Read the model definition and answer for the solid it produces. Units are mm, in the model's axes. Face numbers are marked on the shaded views. A direction names the side the tool comes from. Give positions to 0.01 mm unless a question says otherwise; leave off trailing zeros. Write each loop counter-clockwise with the first axis right and the second up, starting at its lowest first coordinate (ties: lowest second). Pieces come first, ordered by that corner, then holes. Notation, with made-up numbers: (3.5, -5) -> (38.5, -5) arc R15 cw to (38.5, 23) -> close; hole circle Ø11 at (-22, -23.5). An arc over 180 degrees is marked (long way). Write item = value, one per line.
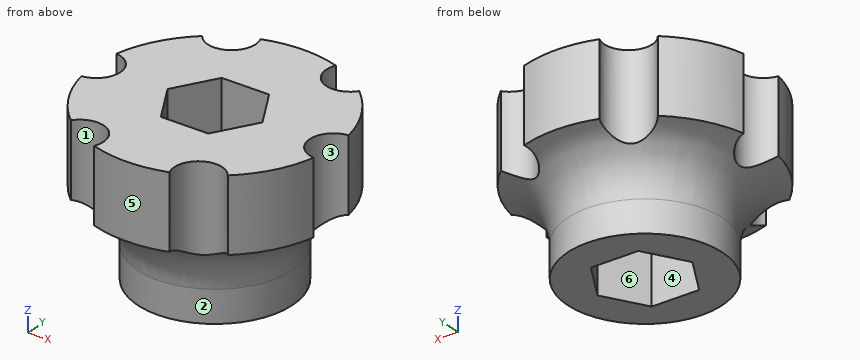
from build123d import *

# Parameters (mm, degrees)
F1_DEPTH = 10


with BuildPart() as f1:
    # F0 (on Top) → F1 (new body)
    with BuildSketch(Plane.XY):
        with BuildLine():
            ThreePointArc((-7.35, 1.492481), (-6, 0), (-7.35, -1.492481))
            ThreePointArc((-7.35, -1.492481), (-6.495191, -3.75), (-4.967527, -5.619046))
            ThreePointArc((-4.967527, -5.619046), (-3, -5.196152), (-2.382473, -7.111527))
            ThreePointArc((-2.382473, -7.111527), (0, -7.5), (2.382473, -7.111527))
            ThreePointArc((2.382473, -7.111527), (3, -5.196152), (4.967527, -5.619046))
            ThreePointArc((4.967527, -5.619046), (6.495191, -3.75), (7.35, -1.492481))
            ThreePointArc((7.35, -1.492481), (6, 0), (7.35, 1.492481))
            ThreePointArc((7.35, 1.492481), (6.495191, 3.75), (4.967527, 5.619046))
            ThreePointArc((4.967527, 5.619046), (3, 5.196152), (2.382473, 7.111527))
            ThreePointArc((2.382473, 7.111527), (0, 7.5), (-2.382473, 7.111527))
            ThreePointArc((-2.382473, 7.111527), (-3, 5.196152), (-4.967527, 5.619046))
            ThreePointArc((-4.967527, 5.619046), (-6.495191, 3.75), (-7.35, 1.492481))
        make_face()
        Polygon((-3.002221, 0), (-1.501111, 2.6), (1.501111, 2.6), (3.002221, 0), (1.501111, -2.6), (-1.501111, -2.6), align=None, mode=Mode.SUBTRACT)
    extrude(amount=F1_DEPTH)

    # F2 (on Front) → F3 (revolve, cut)
    with BuildSketch(Plane.XZ):
        with BuildLine():
            Line((4.85, 2), (4.85, 0))
            Line((4.85, 0), (9.85, 0))
            Line((9.85, 0), (9.924296, 5.125954))
            ThreePointArc((9.924296, 5.125954), (6.514249, 4.979936), (4.85, 2))
        make_face()
    revolve(axis=Axis((0, 0, 4.999244), (0, 0, -1)), mode=Mode.SUBTRACT)


solid = f1.part
(1) The part is cut by section B-B on z = 7.75. Determine the outline of the cut face in (x, y), plus the area to 3 significant figures.
Checks:
outline = (-7.35, -1.49) arc R7.5 ccw to (-4.97, -5.62) arc R1.5 cw to (-2.38, -7.11) arc R7.5 ccw to (2.38, -7.11) arc R1.5 cw to (4.97, -5.62) arc R7.5 ccw to (7.35, -1.49) arc R1.5 cw to (7.35, 1.49) arc R7.5 ccw to (4.97, 5.62) arc R1.5 cw to (2.38, 7.11) arc R7.5 ccw to (-2.38, 7.11) arc R1.5 cw to (-4.97, 5.62) arc R7.5 ccw to (-7.35, 1.49) arc R1.5 cw to start; hole (-3, 0) -> (-1.5, -2.6) -> (1.5, -2.6) -> (3, 0) -> (1.5, 2.6) -> (-1.5, 2.6) -> close
area = 133 mm²
(2) Given P1, Ø1.5, axis at y = 1, z = 2, coming from the +X side; P2, Ø3, axis at y = -0.5, z = 8.5, coming from the -X side; P3, Ø1.5, axis at x = 5.5, z = 7.5, coming from the -Y side, each flat-ended and moving along its own axis, determine where each tip first touches the part or whether it passes through.
Checks:
P1 = 4.87
P2 = -7.35
P3 = -5.62
(3) For a pull along X with two mould halves and no side action, classify the marked faces 1, 2, 3 and 4 as released by +X, released by -X, zero draft, split by the parting line, or undercut.
Checks:
face_1 = undercut
face_2 = split by the parting line
face_3 = released by +X
face_4 = undercut
(4) The part is cut by section C-C on z = 1.75. Determine the outline of the cut face in (x, y).
Checks:
outline = circle Ø9.7 at (0, 0); hole (-3, 0) -> (-1.5, -2.6) -> (1.5, -2.6) -> (3, 0) -> (1.5, 2.6) -> (-1.5, 2.6) -> close
(5) The part is cut by section A-A on x = 0. Determine the outline of the cut face in (y, z).
Checks:
outline = (-7.5, 5.4) arc R3.5 cw to (-4.85, 2) -> (-4.85, 0) -> (-2.6, 0) -> (-2.6, 10) -> (-7.5, 10) -> close; (2.6, 0) -> (4.85, 0) -> (4.85, 2) arc R3.5 cw to (7.5, 5.4) -> (7.5, 10) -> (2.6, 10) -> close
(6) Consider L1, parallel to X at y = 5.5, z = 7.5; L2, parallel to Y at x = 0, z = 9.25; L3, parallel to X at y = 1, z = 4.25. Determine where each line is inside the solid, lowest interval first.
Checks:
L1 = -5.1 to -4.87, -2.63 to 2.63, 4.87 to 5.1
L2 = -7.5 to -2.6, 2.6 to 7.5
L3 = -5.58 to -2.42, 2.42 to 5.58
(7) A tool of negligible diameter and unlimited length cuts with its end or side. For the marked faces 5 and 6, from which of +Z, -Z, +X, -X, +Y, -Y can it reach the whole face along a straight path? Write none if from no direction.
Checks:
face_5 = +Z, -Z, -Y
face_6 = +Z, -Z
(8) The part is cut by section D-D on z = 3.25. Determine the outline of the cut face in (x, y), plus the area to 3 significant figures.
Checks:
outline = circle Ø10.16 at (0, 0); hole (-3, 0) -> (-1.5, -2.6) -> (1.5, -2.6) -> (3, 0) -> (1.5, 2.6) -> (-1.5, 2.6) -> close
area = 57.7 mm²
